Job drawing, mm, ordinate dimensions from the low corner. One solid piece. Give positions to 0.01 mm unless a question says otherwise; leave off trailing zeros. Order: outer loops, then holes, each group sorted by start corner. A loop starts at its lowest first (then second) coordinate and runs counter-clockwise, first axis right, second up. Notation, with made-up numbers: (71, 26.5) - (103, 26.5) arc R18 ccw to (103, 42.5) - close; hole circle Ø11 at (-24.5, 42.5). An arc over 180 degrees is marked (long way). Use one line per item in the form item = value. Start each with the question number.
1. Band-saw the part on B-B, the plane y = 5.25. State how many separate pieces and enclosed holes the cut face has, plus the area to 3 significant figures.
2. Pull direction Y, two halves, no side cores. Call the marked faces 1 and 2: +Y half, -Y half, draft (parallel to the pull), parting line (faces both ways), or undercut.
3. Band-saw the part on A-A, the plane x = 68. List the corners of the cut face in (y, z), plus the area to 3 significant figures.
4. Drill centre lines: line 1 (Z direction, x = 177.8, y = 3); line 2 (X direction, y = 1.5, z = 11) (3 decimals); line 3 (X direction, y = 5.25, z = 47) (3 decimals). Where is each one in solid material? Low to high.
5. Band-saw the part on C-C, the plane x = 128.5. List the corners of the cut face in (y, z).
6. Pin check, flat tips, straight feed: P1, Ø1.9, axis at y = 3, z = 7.5, coming from the -X side; P2, Ø3, axis at y = 2, z = 86, coming from the +X side (3 decimals); P3, Ø1.5, axis at x = 138, y = 1.5, coming from the +Z side. Stop position of each tip, or through.
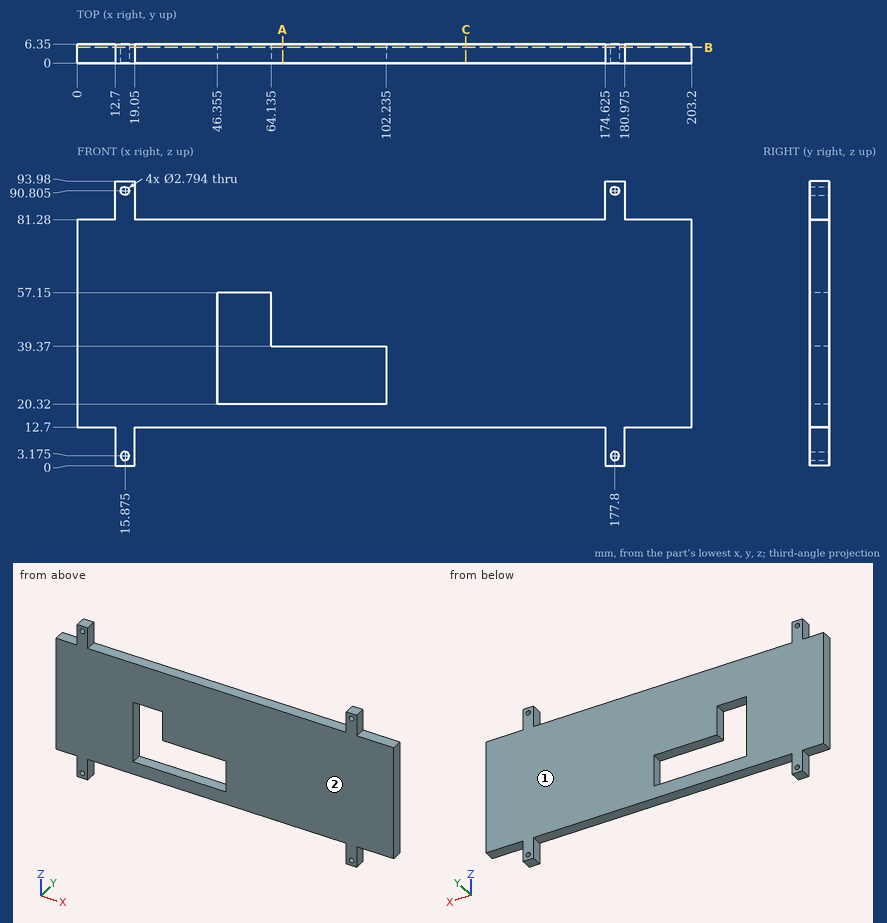
From the geometry:
q1.separate_pieces = 1
q1.enclosed_holes = 5
q1.area = 12,900 mm²
q2.face_1 = +Y half
q2.face_2 = -Y half
q3.outline = (0, 12.7) - (6.35, 12.7) - (6.35, 20.32) - (0, 20.32) - close; (0, 39.37) - (6.35, 39.37) - (6.35, 81.28) - (0, 81.28) - close
q3.area = 315 mm²
q4.line_1 = 0 to 1.78, 4.57 to 89.41, 92.2 to 93.98
q4.line_2 = 12.7 to 19.05, 174.625 to 180.975
q4.line_3 = 0 to 46.355, 64.135 to 203.2
q5.outline = (0, 12.7) - (6.35, 12.7) - (6.35, 81.28) - (0, 81.28) - close
q6.P1 = 12.7
q6.P2 = 180.975
q6.P3 = 81.28
